Input: dimensioned drawing with shaded views. Units: mm. Origin: part minimum x, y, z. A direction names the side the tool comes from. Give positions to 0.01 mm unless a question says otherwise; leave off trailing zeros. Write each loop counter-clockwise with the first axis right and the second up, starting at its lowest first coordinate (ties: lowest second). Pieces come first, ordered by that corner, then holes.
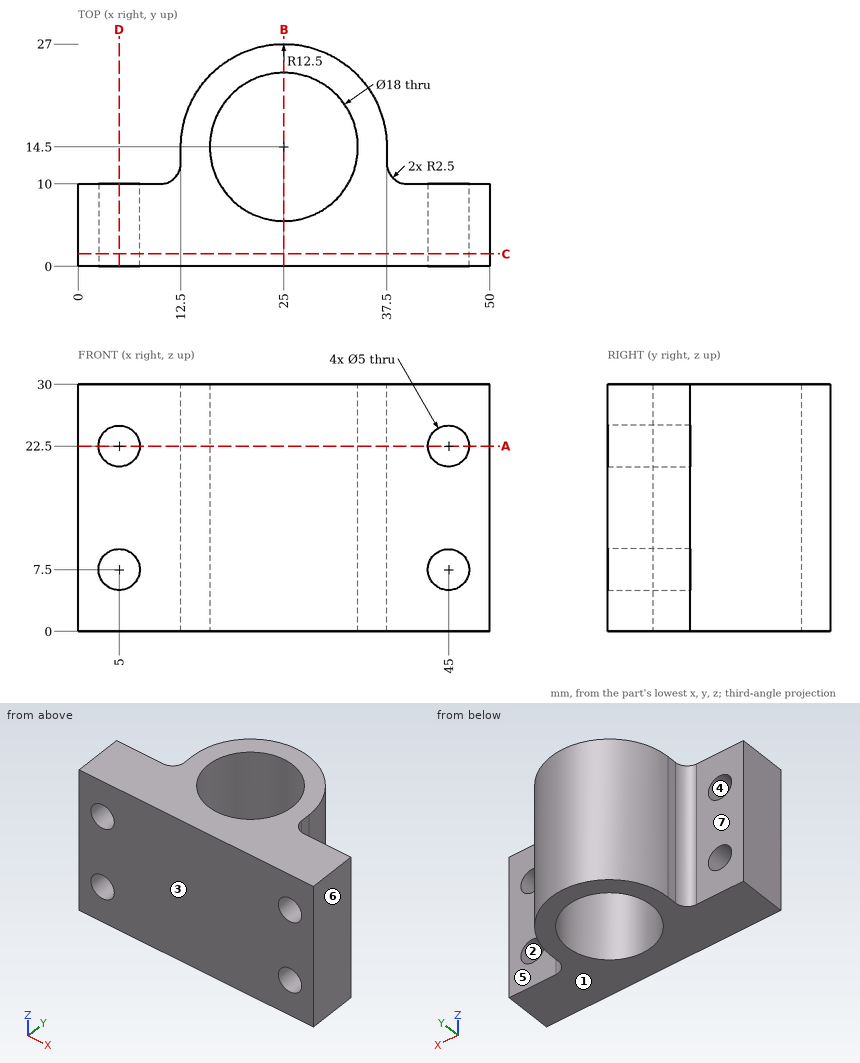
Item 1: Section D-D, the plane x = 5. Return the cut outline in (y, z).
Found:
outline: (0, 0) - (10, 0) - (10, 5) - (0, 5) - close; (0, 10) - (10, 10) - (10, 20) - (0, 20) - close; (0, 25) - (10, 25) - (10, 30) - (0, 30) - close
Item 2: Section A-A, the plane z = 22.5. Return the cut outline in (x, y), plus the area to 3 significant figures.
Found:
outline: (0, 0) - (2.5, 0) - (2.5, 10) - (0, 10) - close; (7.5, 0) - (42.5, 0) - (42.5, 10) - (40, 10) arc R2.5 cw to (37.5, 12.5) - (37.5, 14.5) arc R12.5 ccw to (12.5, 14.5) - (12.5, 12.5) arc R2.5 cw to (10, 10) - (7.5, 10) - close; (47.5, 0) - (50, 0) - (50, 10) - (47.5, 10) - close; hole circle Ø18 at (25, 14.5)
area: 506 mm2
Item 3: Section B-B, the plane x = 25. Return the cut outline in (y, z).
Found:
outline: (0, 0) - (5.5, 0) - (5.5, 30) - (0, 30) - close; (23.5, 0) - (27, 0) - (27, 30) - (23.5, 30) - close
Item 4: Line query: L1, parallel to Y at x = 48, z = 2.25; L2, parallel to X at y = 13.25, z = 18; L3, parallel to Y at x = 24.5, z = 2.5. Output: solid intervals per line, ascending.
Found:
L1: y = 0 to 10
L2: x = 12.5 to 16.09, 33.91 to 37.5
L3: y = 0 to 5.51, 23.49 to 26.99
Item 5: Pull-direction query (Z, two-part tool) for the marked faces 1, 2, 3 and 4; classes: +Z half, -Z half, draft (parallel to the pull), parting line (faces both ways), or undercut.
Found:
face 1: -Z half
face 2: undercut
face 3: draft
face 4: undercut
Item 6: Section C-C, the plane y = 1.5. Return the cut outline in (x, z).
Found:
outline: (0, 0) - (50, 0) - (50, 30) - (0, 30) - close; hole circle Ø5 at (5, 7.5); hole circle Ø5 at (5, 22.5); hole circle Ø5 at (45, 7.5); hole circle Ø5 at (45, 22.5)
Item 7: Pin query (flat end, axial travel): pin 1 Ø6 at (x, y) = (37.5, 13) entering from -Z; pin 2 Ø8 at (y, z) = (19.5, 21.5) entering from -X; pin 3 Ø2 at (x, z) = (34, 21) entering from +Y; pin 4 Ø2 at (y, z) = (14, 12) entering from +X. Return the tip coordinate at first contact, or that it passes through.
Found:
pin 1: stops at z = 0
pin 2: stops at x = 12.54
pin 3: stops at y = 24.1
pin 4: stops at x = 37.5
Item 8: Reachability of the marked faces 5, 6 and 7 from +Z, -Z, +X, -X, +Y, -Y: full face, straight path, thin tool, end or side. Return the list, or none.
Found:
face 5: +Z, -Z, +X, +Y
face 6: +Z, -Z, +X, +Y, -Y
face 7: +Z, -Z, -X, +Y
